Model file for the job. Use its own axes, mm. A direction names the side the tool comes from. Round coordinates to 2 decimals unless told otherwise and drop trailing zeros. Write each loop counter-clockwise with the first axis right and the second up, starting at its lowest first coordinate (ties: lowest second). Pieces come first, ordered by that corner, then holes.
```python
from build123d import *

# Parameters (mm, degrees)
OTHER_10076_5_DEPTH = 0.5
CUT_EXTRUDE1_START  = -0.5
CUT_EXTRUDE1_DEPTH  = 0.5


# Read off the part's stored shape, not the designer's step: 10076-5
with BuildPart() as part:
    # Other 10076-5 outline → Other 10076-5 (new body)
    with BuildSketch(Plane.XY):
        with BuildLine():
            ThreePointArc((7.573674013, -9.436602245), (7.668819519, -9.359444812), (7.763179028, -9.281328104))
            Line((7.763179028, -9.281328104), (7.919995926, -7.488902759))
            ThreePointArc((7.919995926, -7.488902759), (8.548470738, -6.76266575), (9.110578105, -5.983925684))
            ThreePointArc((9.110578105, -5.983925684), (9.242448569, -5.182849851), (8.736493865, -4.547930843))
            Line((8.736493865, -4.547930843), (8.260223146, -4.3))
            Line((8.260223146, -4.3), (5.774945887, -4.3))
            ThreePointArc((5.774945887, -4.3), (5.659072475, -4.451392897), (5.53923133, -4.5996648))
            Line((5.53923133, -4.5996648), (6.59, -6.419649523))
            ThreePointArc((6.59, -6.419649523), (5.831509763, -7.1157216), (5, -7.722693831))
            Line((5, -7.722693831), (5, -7.841555968))
            ThreePointArc((5, -7.841555968), (0, -9.3), (-5, -7.841555968))
            Line((-5, -7.841555968), (-5, -7.722693831))
            ThreePointArc((-5, -7.722693831), (-5.831509763, -7.1157216), (-6.59, -6.419649523))
            Line((-6.59, -6.419649523), (-5.53923133, -4.5996648))
            ThreePointArc((-5.53923133, -4.5996648), (-5.659072475, -4.451392897), (-5.774945887, -4.3))
            Line((-5.774945887, -4.3), (-8.260223146, -4.3))
            Line((-8.260223146, -4.3), (-10.732831081, -5.58715822))
            ThreePointArc((-10.732831081, -5.58715822), (-10.675718173, -5.6955282), (-10.617511084, -5.803314431))
            Line((-10.617511084, -5.803314431), (-9.055174855, -6.258693914))
            ThreePointArc((-9.055174855, -6.258693914), (-8.704696722, -6.64117368), (-8.882127626, -7.128661083))
            Line((-8.882127626, -7.128661083), (-9.436602245, -7.573674013))
            ThreePointArc((-9.436602245, -7.573674013), (-9.359444812, -7.668819519), (-9.281328104, -7.763179028))
            Line((-9.281328104, -7.763179028), (-7.660171598, -7.905011844))
            ThreePointArc((-7.660171598, -7.905011844), (-7.241809703, -8.211767477), (-7.320727248, -8.724502998))
            Line((-7.320727248, -8.724502998), (-7.777730077, -9.269137762))
            ThreePointArc((-7.777730077, -9.269137762), (-7.683493234, -9.347402405), (-7.588468891, -9.424709008))
            Line((-7.588468891, -9.424709008), (-5.970792243, -9.247544602))
            ThreePointArc((-5.970792243, -9.247544602), (-5.500623999, -9.466787654), (-5.477995427, -9.985067155))
            Line((-5.477995427, -9.985067155), (-5.819964104, -10.608393744))
            ThreePointArc((-5.819964104, -10.608393744), (-5.712269322, -10.666769858), (-5.603989074, -10.724052707))
            Line((-5.603989074, -10.724052707), (-4.05195869, -10.234699407))
            ThreePointArc((-4.05195869, -10.234699407), (-3.548052399, -10.358004491), (-3.424747314, -10.861910782))
            Line((-3.424747314, -10.861910782), (-3.638540174, -11.539975104))
            ThreePointArc((-3.638540174, -11.539975104), (-3.521526102, -11.576219327), (-3.404151099, -11.611277074))
            Line((-3.404151099, -11.611277074), (-1.977410637, -10.828540453))
            ThreePointArc((-1.977410637, -10.828540453), (-1.459131136, -10.851169025), (-1.239888083, -11.321337268))
            Line((-1.239888083, -11.321337268), (-1.317289186, -12.028081692))
            ThreePointArc((-1.317289186, -12.028081692), (-1.195452609, -12.04080118), (-1.073493507, -12.052286575))
            Line((-1.073493507, -12.052286575), (0.173128198, -11.006246762))
            ThreePointArc((0.173128198, -11.006246762), (0.685863719, -10.927329218), (0.992619352, -11.345691113))
            Line((0.992619352, -11.345691113), (1.054584487, -12.053955847))
            ThreePointArc((1.054584487, -12.053955847), (1.176561457, -12.042661796), (1.298417839, -12.030133462))
            Line((1.298417839, -12.030133462), (2.317013814, -10.760989181))
            ThreePointArc((2.317013814, -10.760989181), (2.804501216, -10.583558277), (3.186980982, -10.93403641))
            Line((3.186980982, -10.93403641), (3.38593107, -11.616603238))
            ThreePointArc((3.38593107, -11.616603238), (3.503360927, -11.581729673), (3.620431715, -11.545669067))
            Line((3.620431715, -11.545669067), (4.371857887, -10.10219282))
            ThreePointArc((4.371857887, -10.10219282), (4.815363304, -9.833067127), (5.258868721, -10.10219282))
            Line((5.258868721, -10.10219282), (5.58715822, -10.732831081))
            ThreePointArc((5.58715822, -10.732831081), (5.6955282, -10.675718173), (5.803314431, -10.617511084))
            Line((5.803314431, -10.617511084), (6.258693914, -9.055174855))
            ThreePointArc((6.258693914, -9.055174855), (6.64117368, -8.704696722), (7.128661083, -8.882127626))
            Line((7.128661083, -8.882127626), (7.573674013, -9.436602245))
        make_face()
    extrude(amount=OTHER_10076_5_DEPTH)

    # Sketch1 → Cut-Extrude1 (cut)
    with BuildSketch(Plane.XY.offset(0.5).offset(CUT_EXTRUDE1_START)):
        with BuildLine():
            Line((-9.668418082, -5.033059884), (-10.732831081, -5.58715822))
            ThreePointArc((-10.732831081, -5.58715822), (-9.359444812, -7.668819519), (-7.588468891, -9.424709008))
            Line((-7.588468891, -9.424709008), (-5.970792243, -9.247544602))
            ThreePointArc((-5.970792243, -9.247544602), (-5.808080301, -9.256437784), (-5.656869384, -9.317179228))
            ThreePointArc((-5.656869384, -9.317179228), (-7.956414306, -7.450199419), (-9.668418082, -5.033059884))
        make_face()
    extrude(amount=CUT_EXTRUDE1_DEPTH, mode=Mode.SUBTRACT)


solid = part.part
```
1) Cut at C-C on x = -8. List the corners of the cut face in (y, z), and give its area (3 significant figures).
2) Pull direction Y, two halves, no side cores. Call faces 1 (the face through (0.1, -9.3, 0.2)), 2 (the face through (-6.07, -5.52, 0.25)), 3 (the face through (-5.82, -7.125, 0.246)), 4 (the face through (0, -10, 0.5)): released by +Y, released by -Y, zero draft, split by the parting line, or undercut.
3) Cut at B-B on y = -5.25. List the corners of the cut face in (x, z).
4) Which spindle directions (+Z, -Z, +X, -X, +Y, -Y) get a long thin tool onto all of the face, cutting with end or side? Do faces 5 (the face through (-0.46, -11.54, 0.25)), 6 (the face through (0, -10, 0)), 7 (the face through (5.84, -7.11, 0.25)). Say none if no direction does.
5) Wall check: probe 1 along X at (y, z) = (-11, 0.2); probe 2 along X at (y, z) = (-11.25, 0.35); probe 3 along X at (y, z) = (-6, 0.4). Give the ranges that are in metal, low to high.
6) Cut at A-A on y = -8.5. List the corners of the cut face in (x, z), and give its area (3 significant figures).
7) Cut at D-D on x = 2. List the corners of the cut face in (y, z).
Result sheet:
1. outline: (-7.4, 0) - (-4.3, 0) - (-4.3, 0.5) - (-7.4, 0.5) - close
1. area: 1.55 mm2
2. face 1: released by +Y
2. face 2: undercut
2. face 3: undercut
2. face 4: zero draft
3. outline: (-9.55, 0) - (-5.91, 0) - (-5.91, 0.5) - (-9.55, 0.5) - close; (5.91, 0) - (9.26, 0) - (9.26, 0.5) - (5.91, 0.5) - close
4. face 5: +Z, -Z, -Y
4. face 6: -Z, +X, -X, +Y, -Y
4. face 7: +Z, -Z
5. probe 1: x = -3.47 to -2.29, -1.31 to 0.18, 0.81 to 2.13, 3.21 to 3.9
5. probe 2: x = -3.55 to -2.75, -1.24 to -0.12, 0.97 to 1.92, 3.28 to 3.77
5. probe 3: x = -9.1 to -6.35, 6.35 to 9.1
6. outline: (-6.82, 0) - (-3.77, 0) - (-3.77, 0.5) - (-6.82, 0.5) - close; (3.77, 0) - (7.83, 0) - (7.83, 0.5) - (3.77, 0.5) - close
6. area: 3.55 mm2
7. outline: (-11.16, 0) - (-9.08, 0) - (-9.08, 0.5) - (-11.16, 0.5) - close
